Input: part model. Units: mm. Frame: model coordinates. Face numbers are marked on the shaded views. A direction names the side the tool comes from. Give positions to 0.01 mm unless a question says otherwise; leave off trailing zeros. Write each loop counter-clockwise with the first axis right and the second up, starting at its lowest first coordinate (ties: lowest second). Pieces come first, ordered by that corner, then holes. Notation, with made-up numbers: (-27, 78) -> (-16, 78) arc R20 ccw to (-16, 116) -> close; hole circle Ø11 at (25, 79). An arc over 180 degrees is marked (long way). Return JSON: item names as keys, results as strings. Group by question number.
Item 1: Section A-A, the plane z = 6.5. Return loops of the section in (x, y).
Item 2: Pin query (flat end, axial travel): P1, Ø1.5, axis at x = -1.5, y = -6.5, coming from the +Z side; P2, Ø4, axis at x = -2, y = 7.5, coming from the -Z side; P3, Ø2, axis at x = 6.5, y = -7, coming from the -Z side; P4, Ø2.5, axis at x = -2.5, z = 3.5, coming from the -Y side. Return the tip coordinate at first contact, or that it passes through.
Item 3: Section B-B, the plane x = 7.25. Return loops of the section in (y, z), then the cut area to 4 significant figures.
Item 4: Line query: line 1 (Y direction, x = -2.75, z = 4); line 2 (Y direction, x = 5.5, z = 2). Output: solid intervals per line, ascending. Write a range as [from, to].
Item 5: Set-up query: the marked faces 1 and 2. Return all of +Z, -Z, +X, -X, +Y, -Y with unobstructed straight access to the full face (end or side cutting, diameter ignored); none if empty.
Item 6: Section C-C, the plane y = -3.5. Return loops of the section in (x, z).
Item 7: Section D-D, the plane z = 0.75. Return loops of the section in (x, y), then the cut area to 4 significant figures.
from build123d import *

# Parameters (mm, degrees)
F1_DEPTH = 8
F2_SIZE  = 7


with BuildPart() as f1:
    # F0 (on Top) → F1 (new body)
    with BuildSketch(Plane.XY):
        Polygon((10, -10), (10, 10), (-5, 10), (-5, 0), (0, 0), (0, -10), align=None)
    extrude(amount=F1_DEPTH)

    # F2
    f2_edges = [f1.edges().sort_by_distance(p)[0] for p in [
        (5, -10, 0),
    ]]
    chamfer(f2_edges, length=F2_SIZE)


solid = f1.part
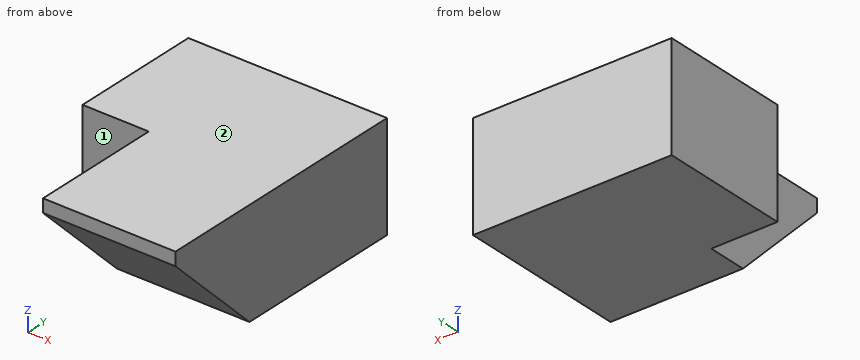
Answer below:
{
 "1": {"outline": "(-5, 0) -> (0, 0) -> (0, -9.5) -> (10, -9.5) -> (10, 10) -> (-5, 10) -> close"},
 "2": {"P1": "passes through", "P2": "stops at z = 0", "P3": "stops at z = 3", "P4": "stops at y = 0"},
 "3": {"outline": "(-10, 7) -> (-3, 0) -> (10, 0) -> (10, 8) -> (-10, 8) -> close", "area": "135.5 mm2"},
 "4": {"line 1": "y = [0, 10]", "line 2": "y = [-5, 10]"},
 "5": {"face 1": "+Z, -Z, -X, -Y", "face 2": "+Z, +X, -X, +Y, -Y"},
 "6": {"outline": "(0, 0.5) -> (10, 0.5) -> (10, 8) -> (0, 8) -> close"},
 "7": {"outline": "(-5, 0) -> (0, 0) -> (0, -3.75) -> (10, -3.75) -> (10, 10) -> (-5, 10) -> close", "area": "187.5 mm2"}
}
